Verification items for the finished model (mm, model axes). Give positions to 0.01 mm unless a question says otherwise; leave off trailing zeros. Use CSV: the item, a comma, the result in double quotes.
from build123d import *

# Parameters (mm, degrees)
BOSS_EXTRUDE5_DEPTH = 1900
SKETCH8_R           = 4.25
CUT_EXTRUDE1_DEPTH  = 9
SKETCH9_R           = 3
CUT_EXTRUDE2_DEPTH  = 12.3
LPATTERN1_COUNT     = 35
LPATTERN1_PITCH     = 60


with BuildPart() as part:
    # Sketch7 → Boss-Extrude5 (new body)
    with BuildSketch(Plane(origin=(58.5, 0, 0), x_dir=(0, 0, -1), z_dir=(1, 0, 0))):
        with BuildLine():
            Line((-7.709038211, 8.883084864), (-8.5, 8.601077183))
            Line((-8.5, 8.601077183), (-8.5, 6.104700538))
            ThreePointArc((-8.5, 6.104700538), (-8.566987298, 5.854700538), (-8.75, 5.671687836))
            Line((-8.75, 5.671687836), (-10, 4.95))
            Line((-10, 4.95), (-10, 1))
            Line((-10, 1), (-9, 0))
            Line((-9, 0), (-4, 0))
            Line((-4, 0), (-3.5, 0.5))
            Line((-3.5, 0.5), (3.5, 0.5))
            Line((3.5, 0.5), (4, 0))
            Line((4, 0), (9, 0))
            Line((9, 0), (10, 1))
            Line((10, 1), (10, 4.95))
            Line((10, 4.95), (8.75, 5.671687836))
            ThreePointArc((8.75, 5.671687836), (8.566987298, 5.854700538), (8.5, 6.104700538))
            Line((8.5, 6.104700538), (8.5, 8.46691323))
            Line((8.5, 8.46691323), (8.084678947, 8.882234283))
            ThreePointArc((8.084678947, 8.882234283), (6.941822875, 9.249266637), (6.503340774, 10.366659226))
            Line((6.503340774, 10.366659226), (6, 10.87))
            Line((6, 10.87), (6, 14.93))
            Line((6, 14.93), (6.503340774, 15.433340774))
            ThreePointArc((6.503340774, 15.433340774), (6.813545517, 16.412959034), (7.709038211, 16.916915136))
            Line((7.709038211, 16.916915136), (8.5, 17.198922817))
            Line((8.5, 17.198922817), (8.5, 19.3))
            Line((8.5, 19.3), (7.5, 20.3))
            Line((7.5, 20.3), (-7.5, 20.3))
            Line((-7.5, 20.3), (-8.5, 19.3))
            Line((-8.5, 19.3), (-8.5, 17.33308677))
            Line((-8.5, 17.33308677), (-8.084678947, 16.917765717))
            ThreePointArc((-8.084678947, 16.917765717), (-6.941822875, 16.550733363), (-6.503340774, 15.433340774))
            Line((-6.503340774, 15.433340774), (-6, 14.93))
            Line((-6, 14.93), (-6, 10.87))
            Line((-6, 10.87), (-6.503340774, 10.366659226))
            ThreePointArc((-6.503340774, 10.366659226), (-6.813545517, 9.387040966), (-7.709038211, 8.883084864))
        make_face()
    extrude(amount=BOSS_EXTRUDE5_DEPTH)

    # Sketch8 → Cut-Extrude1 (cut)
    with BuildSketch(Plane(origin=(0, 20.3, 0), x_dir=(1, 0, 0), z_dir=(0, 1, 0))):
        with Locations((1941.491679108, 0)):
            Circle(SKETCH8_R)
    cut_extrude1 = extrude(amount=-CUT_EXTRUDE1_DEPTH, mode=Mode.SUBTRACT)

    # Sketch9 → Cut-Extrude2 (cut, through all)
    with BuildSketch(Plane(origin=(0, 11.3, 0), x_dir=(1, 0, 0), z_dir=(0, 1, 0))):
        with Locations((1941.491679108, 0)):
            Circle(SKETCH9_R)
    cut_extrude2 = extrude(amount=-CUT_EXTRUDE2_DEPTH, mode=Mode.SUBTRACT)

    # LPattern1: Cut-Extrude1, Cut-Extrude2 ×35
    with Locations(*[(-i * LPATTERN1_PITCH, 0, 0) for i in range(1, LPATTERN1_COUNT)]):
        add(cut_extrude1, mode=Mode.SUBTRACT)
        add(cut_extrude2, mode=Mode.SUBTRACT)


solid = part.part
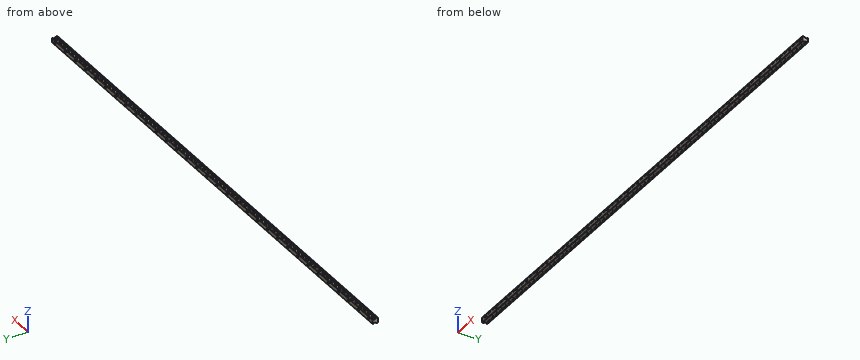
(1) Scan lines: L1, parallel to Z at x = 871.5, y = 16; L2, parallel to Y at x = 737, z = -1.5; L3, parallel to Z at x = 995, y = 16.25. Record each from-to range of solid material in increasing order. Write a range as from..to.
Calculated:
L1,"z = -6.58..6.58"
L2,"y = 0.5..20.3"
L3,"z = -6.7..6.7"
(2) Depth check by flat-ended pin: pin 1 Ø10 at (x, y) = (584.5, 10) entering from -Z; pin 2 Ø5 at (x, z) = (141.49, 0) entering from +Y; pin 3 Ø5 at (x, y) = (1313, 8) entering from +Z; pin 4 Ø10 at (x, y) = (513.5, 9.5) entering from +Z. Enter the tip coordinate at first touch or a pass-through.
Calculated:
pin 1,"stops at z = -9.91"
pin 2,"passes through"
pin 3,"stops at z = 9.05"
pin 4,"stops at z = 10"
(3) Section check B-B on z = 0. Count the separate pieces of the cut face and the enclosed holes in it, plus the area to 3 significant figures.
Calculated:
separate pieces,"33"
enclosed holes,"0"
area,"33,100 mm²"
